Part model, mm, in its own coordinate system. A direction names the side the tool comes from. Give positions to 0.01 mm unless a question says otherwise; leave off trailing zeros. Write each loop counter-clockwise with the first axis right and the second up, starting at its lowest first coordinate (ties: lowest second). Pieces come first, ordered by that corner, then holes. Notation, with made-up numbers: (51, 73.25) - (80, 73.25) arc R34 cw to (80, 112.25) - close; hole circle Ø5 at (-24, 56.25). An arc over 180 degrees is marked (long way). Answer as a JSON object with one key per item and string values. Group by question number.
Autodesk Inventor part; units mm, degrees
ref_plane "Work Plane1" through (5, 0, 0) normal (1, 0, 0) x (0, 1, 0)
ref_plane "Work Plane3" through (13, 5, 0) normal (1, 0, 0) x (0, 0, -1)
ref_plane "Work Plane5" through (13, 4, 1.7321) normal (0, -0.5, 0.8660254) x (1, 0, 0)
sketch "Sketch1" plane through (0, 0, 0) normal (0, 1, 0) x (-1, 0, 0)
  circle A0 centre (0, 0) radius 6
  dimension "d0" = 12
extrude "Extrusion1" add sketch "Sketch1" along normal blind 2
sketch "Sketch2" plane through (0, 2, 0) normal (0, 1, 0) x (1, 0, 0)
  circle A0 centre (0, 0) radius 4
  circle A1 centre (0, 0) radius 6
  dimension "d3" = 8
extrude "Extrusion2" add sketch "Sketch2" along normal blind 33.5
sketch "Sketch3" plane through (0, 35.5, 0) normal (0, 1, 0) x (1, 0, 0)
  arc A0 (-6, 0) -> (0, -6) centre (0, 0) ccw
  circle A1 centre (0, 0) radius 6 construction
  arc A2 (6, 0) -> (0, 6) centre (0, 0) ccw
  line L0 (0, -6) -> (0, -4)
  circle A3 centre (0, 0) radius 4 construction
  line L1 (0, 4) -> (0, 6)
  line L2 (6, 0) -> (4, 0)
  line L3 (-4, 0) -> (-6, 0)
  arc A4 (-4, 0) -> (0, -4) centre (0, 0) ccw
  arc A5 (4, 0) -> (0, 4) centre (0, 0) ccw
extrude "Extrusion3" add sketch "Sketch3" along normal blind 5
ref_plane "Work Plane1" through (5, 0, 0) normal (1, 0, 0) x (0, 1, 0)
sketch "Sketch5" plane through (5, 0, 0) normal (1, 0, 0) x (0, 1, 0)
  line L0 (35.5, 0) -> (35.5, 6) construction
  line L1 (35.5, -6) -> (35.5, 0) construction
  circle A0 centre (5, 0) radius 1.75
  line L2 (0, 6) -> (0, -6)
  line L3 (44.4345, 0) -> (-10, 0) construction
  point P0 (0, 0)
  point P1 (0, 0)
  dimension "d10" = 3.5
  dimension "d44" = 5
extrude "Extrusion4" add sketch "Sketch5" along normal blind 12
pattern_circular "Circular Pattern1" count 3 over 360 about axis through (0, 0, 0) along (0, 1, 0) of "Extrusion4"
thread "Thread1"
thread "Thread2"
thread "Thread3"
ref_plane "Work Plane3" through (13, 5, 0) normal (1, 0, 0) x (0, 0, -1)
sketch "Sketch7" plane through (13, 5, 0) normal (1, 0, 0) x (0, 0, -1)
  circle A0 centre (0, 0) radius 1.75 construction
  arc A1 (0, 6.6281) -> (-5.7401, -3.3141) centre (0, 0) ccw construction
  line L0 (0, 0) -> (-5.7401, -3.3141) construction
  line L1 (0, 0) -> (0, 6.6281) construction
  point P0 (0, -12)
  dimension "d23" = 120
sketch "Sketch8" plane through (0, 0, 0) normal (0, -1, 0) x (1, 0, 0)
  point P0 (0, 0)
  point P1 (0, 0)
hole "Hole1" at (0, 0, 0) direction (0, 1, 0) diameter 2.4 end through all
ref_plane "Work Plane5" through (13, 4, 1.7321) normal (0, -0.5, 0.8660254) x (1, 0, 0)
ref_plane "Work Plane4" through (13, 5, 0) normal (0, -0.5, 0.8660254) x (1, 0, 0)
sketch "Sketch10" plane through (13, 4, 1.7321) normal (0, -0.5, 0.8660254) x (1, 0, 0)
  line L0 (-7, -4.3301) -> (-7, 30.7439) construction
  line L1 (-7, 1.7737) -> (-7, -1.9186) construction
  point P0 (-13, -4.3301)
  point P1 (0, 0)
  dimension "d33" = 7
hole "Hole2" at (13, 4, 1.7321) direction (0, 0.5, -0.8660254) diameter 1 end through all
pattern_circular "Circular Pattern2" count 3 over 360 about axis through (0, 0, 0) along (0, 1, 0) of "Hole2"
properties part number "UntererRührerHalter"
1) Band-saw the part on A-A (y = 37.5). List the corners of the cut face in (x, z), plus the area to 3 significant figures.
2) Mould opens along X. For faces 1 (the cylindrical face through (-6.8, 4.6, -11.3)), 2 (the cylindrical face through (11.29, 3.61, 1.06)), 3 (the flat face through (0, 38, -5)) say: pulls with the +X half, pulls with the -X half, needs draft (parallel to the pull), parting line crosses it, or undercut.
3) Probe line 1 (Z direction, x = 0, y = 1.6); line 2 (Y direction, x = -0.5, z = 3). List the from-to ranges inside material, lowest first.
4) Drop flat-ended pins along their axis: P1, Ø6, axis at x = -1, y = 9.5, coming from the -Z side; P2, Ø0.6, axis at y = 38.5, z = 5, coming from the +X side; P3, Ø4, axis at y = 32.5, z = 1, coming from the -X side; P4, Ø6.5, axis at x = -2, z = -4, coming from the +Y side. Give the stop position or say it passes through.
5) Which spindle directions (+Z, -Z, +X, -X, +Y, -Y) get a long thin tool onto all of the face, cutting with end or side? Do faces 4 (the flat face through (1, 2, -1)), 5 (the flat face through (3, 35.5, 3)), 6 (the flat face through (-5, 38, 0)). Say none if no direction does.
6) Band-saw the part on B-B (y = 29). List the corners of the cut face in (x, z), plus the area to 3 significant figures.
7) Band-saw the part on C-C (x = 11.75). List the corners of the cut face in (y, z).
Verdict:
{
 "1": {"outline": "(-6, 0) - (-4, 0) arc R4 cw to (0, 4) - (0, 6) arc R6 ccw to start; (0, -6) arc R6 ccw to (6, 0) - (4, 0) arc R4 cw to (0, -4) - close", "area": "31.4 mm2"},
 "2": {"face 1": "undercut", "face 2": "needs draft", "face 3": "pulls with the -X half"},
 "3": {"line 1": "-6 to -1.2, 1.2 to 6", "line 2": "0 to 2"},
 "4": {"P1": "z = -6", "P2": "x = 0", "P3": "x = -6", "P4": "y = 40.5"},
 "5": {"face 4": "+Y", "face 5": "+Z, +X, +Y", "face 6": "-Z, -X, +Y"},
 "6": {"outline": "circle Ø12 at (0, 0); hole circle Ø8 at (0, 0)", "area": "62.8 mm2"},
 "7": {"outline": "circle Ø3.5 at (5, 0)"}
}
